The listing builds one solid part. Answer for the finished solid, in the listing's coordinates (mm). Face numbers are marked on the shaded views. A direction names the side the tool comes from. Coordinates: 2 decimals unless noted, no trailing zeros. Loops run counter-clockwise (first coordinate to the right, second up) from the corner with the lowest first, then second, coordinate; pieces in that order, holes last. Notation, with made-up numbers: (15, 77) - (68, 77) arc R22 ccw to (68, 86) - close; hole circle Ø1 at (22, -28). An arc over 180 degrees is marked (long way). One line per question, with ' | ' between items.
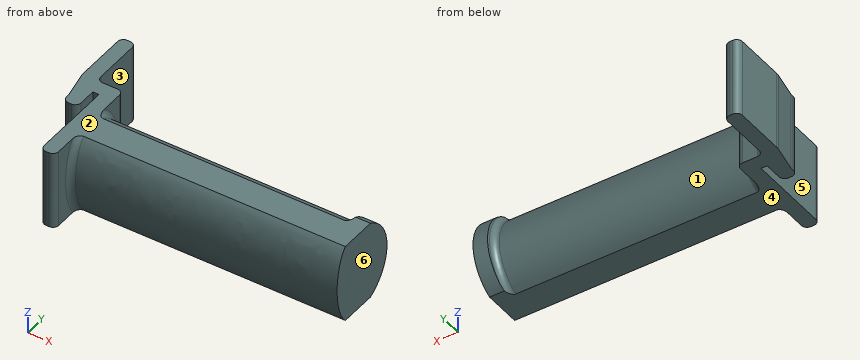
from build123d import *

# Parameters (mm, degrees)
F3_DEPTH = 13.5
F5_DEPTH = 92
F7_DEPTH = 5
F8_R     = 2


with BuildPart() as f3:
    # F2 (on Top) → F3 (new body, symmetric)
    with BuildSketch(Plane.XY):
        with BuildLine():
            ThreePointArc((-12.1, -11), (-11.5142135624, -12.4142135624), (-10.1, -13))
            Line((-10.1, -13), (-9.1, -13))
            ThreePointArc((-9.1, -13), (-7.6857864376, -12.4142135624), (-7.1, -11))
            Line((-7.1, -11), (-7.1, -5))
            Line((-7.1, -5), (-5, -5))
            Line((-5, -5), (-5, -33))
            ThreePointArc((-5, -33), (-4.4142135624, -34.4142135624), (-3, -35))
            Line((-3, -35), (-2, -35))
            ThreePointArc((-2, -35), (-0.5857864376, -34.4142135624), (0, -33))
            Line((0, -33), (0, -2))
            ThreePointArc((0, -2), (-0.5857864376, -0.5857864376), (-2, 0))
            Line((-2, 0), (-7.1, 0))
            ThreePointArc((-7.1, 0), (-8.5142135624, 0.5857864376), (-9.1, 2))
            Line((-9.1, 2), (-9.1, 18))
            ThreePointArc((-9.1, 18), (-9.6857864376, 19.4142135624), (-11.1, 20))
            Line((-11.1, 20), (-12.1, 20))
            ThreePointArc((-12.1, 20), (-13.5142135624, 19.4142135624), (-14.1, 18))
            Line((-14.1, 18), (-14.1, 0.495097568))
            ThreePointArc((-14.1, 0.495097568), (-14.0756666333, 0.0024094781), (-14.0029033785, -0.4854831077))
            Line((-14.0029033785, -0.4854831077), (-12.1970966215, -9.5145168923))
            ThreePointArc((-12.1970966215, -9.5145168923), (-12.1243333667, -10.0024094781), (-12.1, -10.495097568))
            Line((-12.1, -10.495097568), (-12.1, -11))
        make_face()
    extrude(amount=F3_DEPTH, both=True)

    # F4 (on face) → F5 (join)
    with BuildSketch(Plane.YZ):
        with BuildLine():
            Line((-23.2691742077, -13.5), (-16.7308257923, -13.5))
            add(Edge.make_bspline(
                [(-16.7308257923, -13.5), (-2.7938199597, 0), (-16.7308257923, 13.5)],
                knots=[0.4510268118, 0.4510268118, 0.4510268118, 2.6905658418, 2.6905658418, 2.6905658418], degree=2, weights=[1, 0.4358898944, 1]))
            Line((-16.7308257923, 13.5), (-23.2691742077, 13.5))
            add(Edge.make_bspline(
                [(-23.2691742077, 13.5), (-37.2061800403, 0), (-23.2691742077, -13.5)],
                knots=[3.5926194654, 3.5926194654, 3.5926194654, 5.8321584954, 5.8321584954, 5.8321584954], degree=2, weights=[1, 0.4358898944, 1]))
        make_face()
        with BuildLine():
            Line((-16.7308257923, -13.5), (-13.4616515847, -13.5))
            ThreePointArc((-13.4616515847, -13.5), (-5, 0), (-13.4616515847, 13.5))
            Line((-13.4616515847, 13.5), (-16.7308257923, 13.5))
            add(Edge.make_bspline(
                [(-16.7308257923, -13.5), (-2.7938199597, 0), (-16.7308257923, 13.5)],
                knots=[0.4510268118, 0.4510268118, 0.4510268118, 2.6905658418, 2.6905658418, 2.6905658418], degree=2, weights=[1, 0.4358898944, 1]))
        make_face()
    extrude(amount=F5_DEPTH)

    # F6 (on face) → F7 (join)
    with BuildSketch(Plane.YZ.offset(92)):
        with BuildLine():
            Line((-10.4616515847, 13.5), (-13.4616515847, 13.5))
            ThreePointArc((-13.4616515847, 13.5), (-5, 0), (-13.4616515847, -13.5))
            Line((-13.4616515847, -13.5), (-10.4616515847, -13.5))
            ThreePointArc((-10.4616515847, -13.5), (-2, 0), (-10.4616515847, 13.5))
        make_face()
    extrude(amount=-F7_DEPTH)

    # F8
    f8_edges = [f3.edges().sort_by_distance(p)[0] for p in [
        (0, -5, 0),
        (0, -27.5, -0.000816),
        (87, -5, 0),
    ]]
    fillet(f8_edges, radius=F8_R)


solid = f3.part
Item 1: Find the intervals of material crossed by line 1 (X direction, y = -10.5, z = -6.5); line 2 (Y direction, x = 79, z = -0.25); line 3 (X direction, y = -16.5, z = -3), in increasing order. Write a range as [from, to].
Taken from the geometry:
line 1: x = [-12.1, -7.1], [-5, 92] | line 2: y = [-27.5, -5] | line 3: x = [-5, 92]
Item 2: Each of these flat-tipped pins is pushed along its axis until it touches: pin 1 Ø1.7 at (y, z) = (-3.5, -1) entering from -X; pin 2 Ø10 at (x, z) = (10, 1) entering from -Y; pin 3 Ø4 at (x, z) = (20.5, -4.5) entering from -Y. Where does it stop, or does it pass through?
Taken from the geometry:
pin 1: stops at x = -13.57 | pin 2: stops at y = -27.5 | pin 3: stops at y = -27.4
Item 3: Find section A-A, the plane y = -18.5. Write down the section's boundary in (x, z).
Taken from the geometry:
outline: (-5, -13.5) - (92, -13.5) - (92, 13.5) - (-5, 13.5) - close
Item 4: The mould has two halves that part along X. Classify the marked faces 4, 5 and 6: pulls with the +X half, pulls with the -X half, needs draft (parallel to the pull), parting line crosses it, or undercut.
Taken from the geometry:
face 4: needs draft | face 5: undercut | face 6: pulls with the +X half
Item 5: Find section B-B, the plane x = -1. Write down the section's boundary in (y, z).
Taken from the geometry:
outline: (-34.73, -13.5) - (-0.27, -13.5) - (-0.27, 13.5) - (-34.73, 13.5) - close
Item 6: Which of the six approach directions +Z, -Z, +X, -X, +Y, -Y give full straight-line access (tool end or side, diameter ignored) to the marked faces 1, 2 and 3?
Taken from the geometry:
face 1: +Y | face 2: +Z, +X, -X, +Y, -Y | face 3: +Z, -Z, +X, +Y
